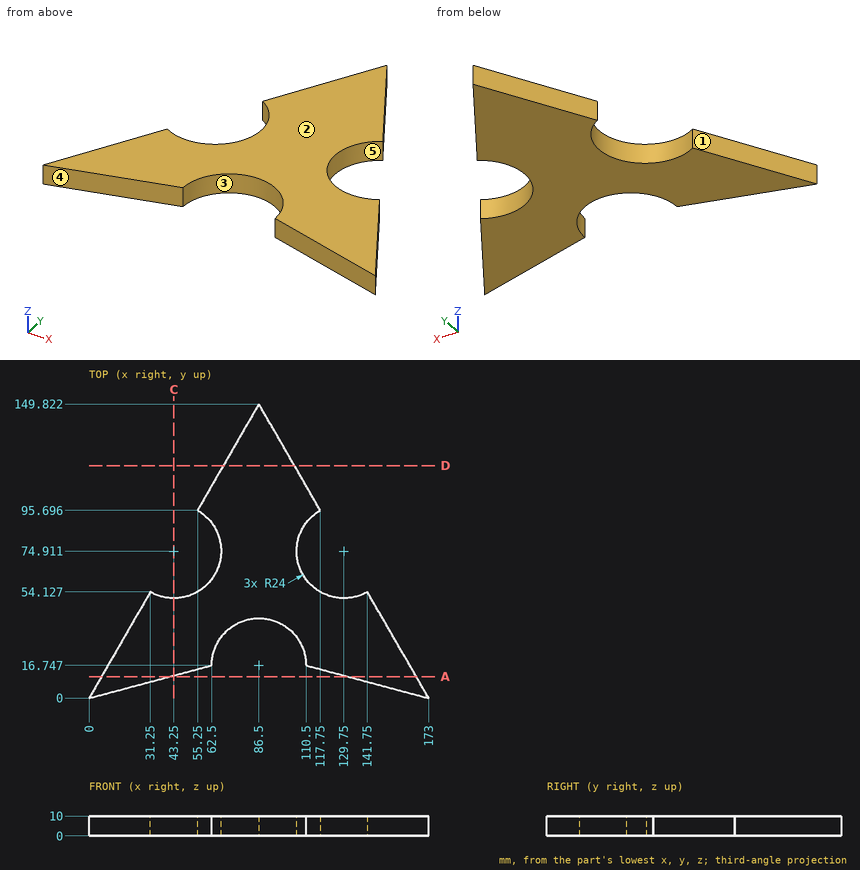
Geometry: see drawing. Coordinates: mm, zero at the bounding-box minimum. A direction names the side the tool comes from. Give positions to 0.01 mm unless a question says otherwise; leave off trailing zeros. Loops run counter-clockwise (first coordinate to the right, second up) from the corner with the lowest first, then second, coordinate; pieces in that order, holes last. Notation, with made-up numbers: (-39.5, 38) - (-34.5, 38) arc R26 ccw to (-34.5, 55) - close; hole circle Ø7 at (41.5, 9). An arc over 180 degrees is marked (long way). Use CSV: the item, a comma, the result in double quotes. Start each with the question number.
Item 1: Contact query for flat-ended pins moving along their axis: P1, Ø12, axis at x = 82.5, y = 106.5, coming from the -Z side; P2, Ø4, axis at y = 42, z = 2, coming from the -X side (1 decimal); P3, Ø2, axis at x = 111.5, z = 4.5, coming from the -Y side; P4, Ø1, axis at y = 86.5, z = 8, coming from the +X side. Output: stop coordinate, or through.
Item 2: Section C-C on x = 43.25. Return loops of the section in (y, z), then the cut area to 3 significant figures.
Item 3: Reachability of the marked faces 4 and 5 from +Z, -Z, +X, -X, +Y, -Y: full face, straight path, thin tool, end or side. Return the list, or none.
Item 4: Mould query, pull axis X, two halves, no side actions, for the marked faces 1, 2 and 3. Classes: pulls with the +X half, pulls with the -X half, needs draft (parallel to the pull), parting line crosses it, or undercut.
Item 5: Section A-A on y = 11. Return loops of the section in (x, z).
Item 6: Line query: line 1 (Y direction, x = 57, z = 4.75) (1 decimal); line 2 (X direction, y = 80.5, z = 5.5); line 3 (X direction, y = 41, z = 8.5). Output: solid intervals per line, ascending.
Item 7: Section D-D on y = 118.5. Return loops of the section in (x, z), then the cut area to 3 significant figures.
Ans:
1,P1,"stops at z = 0"
1,P2,"stops at x = 23.1"
1,P3,"stops at y = 16.21"
1,P4,"stops at x = 109.02"
2,outline,"(11.59, 0) - (50.91, 0) - (50.91, 10) - (11.59, 10) - close"
2,area,"393 mm2"
3,face 4,"+Z, -Z, -Y"
3,face 5,"+Z, -Z"
4,face 1,"pulls with the -X half"
4,face 2,"needs draft"
4,face 3,"undercut"
5,outline,"(6.35, 0) - (41.05, 0) - (41.05, 10) - (6.35, 10) - close; (131.95, 0) - (166.65, 0) - (166.65, 10) - (131.95, 10) - close"
6,line 1,"y = 15.3 to 55.2, 94.6 to 98.7"
6,line 2,"x = 66.59 to 106.41"
6,line 3,"x = 23.67 to 149.33"
7,outline,"(68.42, 0) - (104.58, 0) - (104.58, 10) - (68.42, 10) - close"
7,area,"362 mm2"
